Design review of the part built by this model. Coordinates are the model's own, in mm. A direction names the side the tool comes from. Round coordinates to 2 decimals unless told otherwise and drop trailing zeros. Order: outer loops, then holes, each group sorted by start corner. A loop starts at its lowest first (then second) coordinate and runs counter-clockwise, first axis right, second up. Notation, with made-up numbers: M -37.75,40 L -7.75,40 A26 ccw -7.75,59 Z; hole C -33.5,36 d8. An arc over 180 degrees is marked long. Write each question's results on one line, items separated by ' | '. Start each with the question number.
Item 1: Machinability: for faces 4 (the flat face through (31.615, 5.07, -85.781)), 5 (the flat face through (19, 0, -45)), which of the approach directions +Z, -Z, +X, -X, +Y, -Y give a long, thin tool a straight path to every point of the face, cutting with its end or side? Answer none if there is none.
Item 2: Take a section at A-A, the plane z = 0. Write out the cut boundary in (x, y).
Item 3: Clearance check with flat-ended pins moving along their axes: pin 1 (1.5 mm diameter, centred on y = 9, z = -47, fed in from +X); pin 2 (6 mm diameter, centred on x = -26.5, y = 2, fed in from -Z); pin 3 (6 mm diameter, centred on x = -6, y = 7.5, fed in from +Z). State where each tip first meets the part, or that it passes through.
Item 4: The part is to be moulded in two halves that separate along X. For faces 1 (the flat face through (34.817, 5.07, -77.228)), 2 (the cylindrical face through (-11.24, 5.07, -11.21)), 3 (the flat face through (22.634, 4.93, -36.899)), say which applies: +X half, -X half, draft (parallel to the pull), parting line (faces both ways), or undercut.
Item 5: Wall thickness on line 1 (Z direction, x = 0, y = 4.5); line 2 (X direction, y = 4.25, z = 0); line 3 (Z direction, x = 5.5, y = 2): over which ranges is each line inside the solid? List them lowest first. Write a range as [from, to].
Item 6: Take a section at B-B, the plane x = 0. Write out the cut boundary in (y, z), plus the area to 3 significant figures.
```python
from build123d import *

# Parameters (mm, degrees)
BOSS_EXTRUDE1_DEPTH = 10
FILLET1_R           = 5
CUT_EXTRUDE1_DEPTH  = 121.593129692
FILLET2_R           = 0.5


with BuildPart() as part:
    # Sketch1 → Boss-Extrude1 (new body)
    with BuildSketch(Plane(origin=(0, 0, 0), x_dir=(1, 0, 0), z_dir=(0, 1, 0))):
        with BuildLine():
            Line((10.30016758, 10.9044279), (33.8799835, 60.602564318))
            ThreePointArc((33.8799835, 60.602564318), (0, 114.177287273), (-33.8799835, 60.602564318))
            Line((-33.8799835, 60.602564318), (-10.30016758, 10.9044279))
            ThreePointArc((-10.30016758, 10.9044279), (0, -15), (10.30016758, 10.9044279))
        make_face()
        with BuildLine():
            Line((27.1039868, 63.817508909), (1.514929585, 9.884583368))
            ThreePointArc((1.514929585, 9.884583368), (0, -10), (-1.514929585, 9.884583368))
            Line((-1.514929585, 9.884583368), (-27.1039868, 63.817508909))
            ThreePointArc((-27.1039868, 63.817508909), (0, 106.677287273), (27.1039868, 63.817508909))
        make_face(mode=Mode.SUBTRACT)
    extrude(amount=BOSS_EXTRUDE1_DEPTH)

    # Fillet1
    fillet1_edges = [part.edges().sort_by_distance(p)[0] for p in [
        (10.30016758, 5, -10.9044279),
        (-10.30016758, 5, -10.9044279),
        (1.514929585, 5, -9.884583368),
        (-1.514929585, 5, -9.884583368),
    ]]
    fillet(fillet1_edges, radius=FILLET1_R)

    # Sketch2 → Cut-Extrude1 (cut, through all)
    with BuildSketch(Plane(origin=(0, 10, 0), x_dir=(1, 0, 0), z_dir=(0, 1, 0))):
        with BuildLine():
            Line((21.877604248, 88.906739184), (34.135902296, 84.971177619))
            ThreePointArc((34.135902296, 84.971177619), (34.387053168, 84.789711637), (34.483059832, 84.495111257))
            Line((34.483059832, 84.495111257), (34.483059832, 82.414608392))
            ThreePointArc((34.483059832, 82.414608392), (34.398003238, 82.135642498), (34.171771953, 81.95158816))
            Line((34.171771953, 81.95158816), (32.294347711, 81.186410559))
            ThreePointArc((32.294347711, 81.186410559), (32.068116426, 81.00235622), (31.983059832, 80.723390327))
            Line((31.983059832, 80.723390327), (31.983059832, 78.082279644))
            ThreePointArc((31.983059832, 78.082279644), (32.079066495, 77.787679264), (32.330217368, 77.606213282))
            Line((32.330217368, 77.606213282), (46.132813135, 73.174850528))
            Line((46.132813135, 73.174850528), (46.255087106, 73.555703617))
            Line((46.255087106, 73.555703617), (32.730217368, 77.897901638))
            ThreePointArc((32.730217368, 77.897901638), (32.479066495, 78.07936762), (32.383059832, 78.373968))
            Line((32.383059832, 78.373968), (32.383059832, 80.454470865))
            ThreePointArc((32.383059832, 80.454470865), (32.468116426, 80.733436759), (32.694347711, 80.917491097))
            Line((32.694347711, 80.917491097), (34.571771953, 81.682668698))
            ThreePointArc((34.571771953, 81.682668698), (34.798003238, 81.866723036), (34.883059832, 82.14568893))
            Line((34.883059832, 82.14568893), (34.883059832, 84.786799612))
            ThreePointArc((34.883059832, 84.786799612), (34.787053168, 85.081399993), (34.535902296, 85.262865975))
            Line((34.535902296, 85.262865975), (21.999878219, 89.287592274))
            Line((21.999878219, 89.287592274), (21.877604248, 88.906739184))
        make_face()
    extrude(amount=-CUT_EXTRUDE1_DEPTH, mode=Mode.SUBTRACT)

    # Fillet2
    fillet2_edges = [part.edges().sort_by_distance(p)[0] for p in [
        (28.037681738, 5, -87.349138226),
        (37.498715951, 5, -76.366961562),
        (37.492921713, 5, -75.948712321),
        (28.214590334, 5, -86.87223172),
    ]]
    fillet(fillet2_edges, radius=FILLET2_R)


solid = part.part
```
Results list:
1) face 4: +Y, -Y | face 5: +Z, -Z, +X, -X, -Y
2) outline: M -15,0 L -10,0 L -10,10 L -15,10 Z; M 10,0 L 15,0 L 15,10 L 10,10 Z
3) pin 1: x = 27.78 | pin 2: z = -105.9 | pin 3: z = 14.7
4) face 1: undercut | face 2: -X half | face 3: +X half
5) line 1: [-114.18, -106.68], [10, 15] | line 2: [-15, -10], [10, 15] | line 3: [-113.77, -106.17], [-18.28, -8.35], [8.35, 13.96]
6) outline: M 0,-114.18 L 10,-114.18 L 10,-106.68 L 0,-106.68 Z; M 0,10 L 10,10 L 10,15 L 0,15 Z | area: 125 mm²
